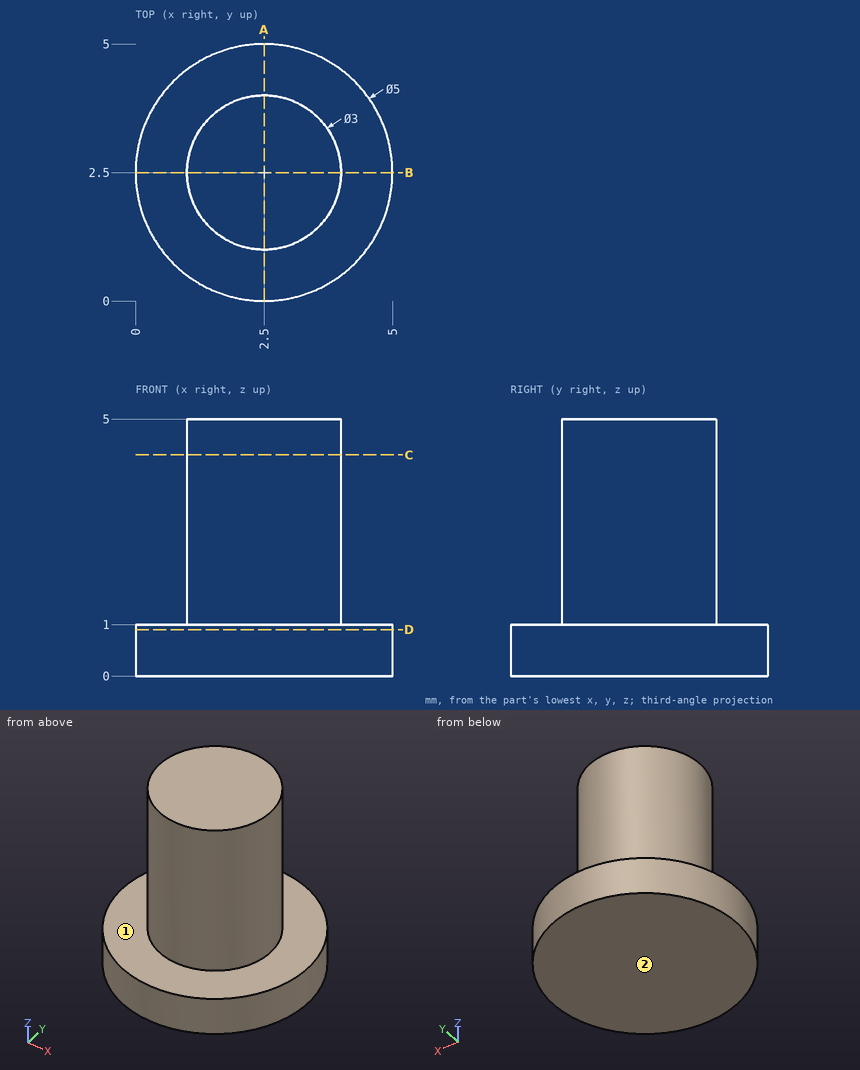
Answer from the drawing. Dimensions are ordinates in mm from the lowest x, y and z of the part. A direction names the side the tool comes from. Coordinates: 2 decimals unless noted, no trailing zeros. Loops run counter-clockwise (first coordinate to the right, second up) from the corner with the lowest first, then second, coordinate; pieces in that order, holes last. Notation, with made-up numbers: (86, 2.25) -> (139, 2.25) arc R26 ccw to (139, 21.25) -> close; hole circle Ø1 at (7, 60). An arc over 180 degrees is marked (long way). Answer as CSV lines item,"result".
Q1. A tool of negligible diameter and unlimited length cuts with its end or side. For the marked faces 1 and 2, from which of +Z, -Z, +X, -X, +Y, -Y can it reach the whole face along a straight path? Write none if from no direction.
Findings:
face 1,"+Z"
face 2,"-Z, +X, -X, +Y, -Y"
Q2. Find the intervals of material crossed by probe 1 along Z at (x, y) = (4.05, 2.6); probe 2 along Y at (x, z) = (3.35, 0.3); probe 3 along X at (y, z) = (2.2, 1.55), in increasing order.
Findings:
probe 1,"z = 0 to 1"
probe 2,"y = 0.15 to 4.85"
probe 3,"x = 1.03 to 3.97"
Q3. The part is cut by section D-D on z = 0.9. Write down the section's boundary in (x, y).
Findings:
outline,"circle Ø5 at (2.5, 2.5)"
Q4. The part is cut by section C-C on z = 4.3. Write down the section's boundary in (x, y), and give its area (3 significant figures).
Findings:
outline,"circle Ø3 at (2.5, 2.5)"
area,"7.07 mm²"
Q5. The part is cut by section A-A on x = 2.5. Write down the section's boundary in (y, z).
Findings:
outline,"(0, 0) -> (5, 0) -> (5, 1) -> (4, 1) -> (4, 5) -> (1, 5) -> (1, 1) -> (0, 1) -> close"
